```python
from build123d import *

# Parameters (mm, degrees)
EXTRUDE1_DEPTH                 = 2.515
M3X0_5_TAPPED_HOLE2_AT_2_COUNT = 2
M3X0_5_TAPPED_HOLE2_AT_2_PITCH = 37
M3X0_5_TAPPED_HOLE2_AT_3_COUNT = 2
M3X0_5_TAPPED_HOLE2_AT_3_PITCH = 74
M3X0_5_TAPPED_HOLE2_AT_4_COUNT = 2
M3X0_5_TAPPED_HOLE2_AT_4_PITCH = 111
M3X0_5_TAPPED_HOLE2_AT_5_COUNT = 2
M3X0_5_TAPPED_HOLE2_AT_5_PITCH = 148
CUT_EXTRUDE1_DEPTH             = 6.03
M3X0_5_TAPPED_HOLE1_D          = 3
M3X0_5_TAPPED_HOLE1_DEPTH      = 7.5
M3X0_5_TAPPED_HOLE1_TIP        = 0.901290929
F_2_5_2_5_DIAMETER_HOLE1_D     = 2.5
F_2_5_2_5_DIAMETER_HOLE1_DEPTH = 6
F_2_5_2_5_DIAMETER_HOLE1_TIP   = 0.751075774


with BuildPart() as part:
    # Sketch1 → Extrude1 (new body, symmetric)
    with BuildSketch(Plane.XY):
        with BuildLine():
            Line((29.232493618, 208), (4.5, 208))
            Line((4.5, 208), (4.5, 37.873672337))
            ThreePointArc((4.5, 37.873672337), (38.14007153, 0), (4.5, -37.873672337))
            Line((4.5, -37.873672337), (4.5, -208))
            Line((4.5, -208), (29.232493618, -208))
            Line((29.232493618, -208), (12, -85.384436669))
            Line((12, -85.384436669), (12, -60))
            ThreePointArc((12, -60), (14.850141486, -49.710084891), (22.588235294, -42.352941176))
            ThreePointArc((22.588235294, -42.352941176), (48, 0), (22.588235294, 42.352941176))
            ThreePointArc((22.588235294, 42.352941176), (14.850141486, 49.710084891), (12, 60))
            Line((12, 60), (12, 85.384436669))
            Line((12, 85.384436669), (29.232493618, 208))
        make_face()
    extrude(amount=EXTRUDE1_DEPTH, both=True)

    # Sketch32 → M3x0.5 Tapped Hole2 (revolve, cut)
    with BuildSketch(Plane(origin=(4.5, 198, 0), x_dir=(0, 0, 1), z_dir=(0, 1, 0))):
        Polygon((0, 0), (0, 8.401290929), (1.5, 7.5), (1.5, 0), align=None)
    m3x0_5_tapped_hole2 = revolve(axis=Axis((-1.85, 198, 0), (1, 0, 0)), mode=Mode.SUBTRACT)

    # M3x0.5 Tapped Hole2 at 2: M3x0.5 Tapped Hole2 ×2
    with Locations(*[(0, -i * M3X0_5_TAPPED_HOLE2_AT_2_PITCH, 0) for i in range(1, M3X0_5_TAPPED_HOLE2_AT_2_COUNT)]):
        add(m3x0_5_tapped_hole2, mode=Mode.SUBTRACT)

    # M3x0.5 Tapped Hole2 at 3: M3x0.5 Tapped Hole2 ×2
    with Locations(*[(0, -i * M3X0_5_TAPPED_HOLE2_AT_3_PITCH, 0) for i in range(1, M3X0_5_TAPPED_HOLE2_AT_3_COUNT)]):
        add(m3x0_5_tapped_hole2, mode=Mode.SUBTRACT)

    # M3x0.5 Tapped Hole2 at 4: M3x0.5 Tapped Hole2 ×2
    with Locations(*[(0, -i * M3X0_5_TAPPED_HOLE2_AT_4_PITCH, 0) for i in range(1, M3X0_5_TAPPED_HOLE2_AT_4_COUNT)]):
        add(m3x0_5_tapped_hole2, mode=Mode.SUBTRACT)

    # M3x0.5 Tapped Hole2 at 5: M3x0.5 Tapped Hole2 ×2
    with Locations(*[(0, -i * M3X0_5_TAPPED_HOLE2_AT_5_PITCH, 0) for i in range(1, M3X0_5_TAPPED_HOLE2_AT_5_COUNT)]):
        add(m3x0_5_tapped_hole2, mode=Mode.SUBTRACT)

    # Mirror2: M3x0.5 Tapped Hole2 across plane
    add(m3x0_5_tapped_hole2.mirror(Plane.ZX), mode=Mode.SUBTRACT)

    # Mirror2 copy 1 sketch → Mirror2 copy 1 (revolve, cut)
    with BuildSketch(Plane(origin=(4.5, -161, 0), x_dir=(0, 0, 1), z_dir=(0, -1, 0))):
        Polygon((0, 0), (0, -8.401290929), (1.5, -7.5), (1.5, 0), align=None)
    revolve(axis=Axis((-1.85, -161, 0), (-1, 0, 0)), mode=Mode.SUBTRACT)

    # Mirror2 copy 2 sketch → Mirror2 copy 2 (revolve, cut)
    with BuildSketch(Plane(origin=(4.5, -124, 0), x_dir=(0, 0, 1), z_dir=(0, -1, 0))):
        Polygon((0, 0), (0, -8.401290929), (1.5, -7.5), (1.5, 0), align=None)
    revolve(axis=Axis((-1.85, -124, 0), (-1, 0, 0)), mode=Mode.SUBTRACT)

    # Mirror2 copy 3 sketch → Mirror2 copy 3 (revolve, cut)
    with BuildSketch(Plane(origin=(4.5, -87, 0), x_dir=(0, 0, 1), z_dir=(0, -1, 0))):
        Polygon((0, 0), (0, -8.401290929), (1.5, -7.5), (1.5, 0), align=None)
    revolve(axis=Axis((-1.85, -87, 0), (-1, 0, 0)), mode=Mode.SUBTRACT)

    # Mirror2 copy 4 sketch → Mirror2 copy 4 (revolve, cut)
    with BuildSketch(Plane(origin=(4.5, -50, 0), x_dir=(0, 0, 1), z_dir=(0, -1, 0))):
        Polygon((0, 0), (0, -8.401290929), (1.5, -7.5), (1.5, 0), align=None)
    revolve(axis=Axis((-1.85, -50, 0), (-1, 0, 0)), mode=Mode.SUBTRACT)

    # Sketch36 → Cut-Extrude1 (cut, through all)
    with BuildSketch(Plane.XY.offset(2.515)):
        with BuildLine():
            Line((4.5, 193), (27.124381098, 193))
            Line((27.124381098, 193), (12, 85.384436669))
            Line((12, 85.384436669), (12, 60))
            ThreePointArc((12, 60), (14.850141486, 49.710084891), (22.588235294, 42.352941176))
            ThreePointArc((22.588235294, 42.352941176), (48, 0), (22.588235294, -42.352941176))
            ThreePointArc((22.588235294, -42.352941176), (14.850141486, -49.710084891), (12, -60))
            Line((12, -60), (12, -85.384436669))
            Line((12, -85.384436669), (29.232493618, -208))
            Line((29.232493618, -208), (4.5, -208))
            Line((4.5, -208), (4.5, -37.873672337))
            ThreePointArc((4.5, -37.873672337), (38.14007153, 0), (4.5, 37.873672337))
            Line((4.5, 37.873672337), (4.5, 193))
        make_face()
    extrude(amount=-CUT_EXTRUDE1_DEPTH, mode=Mode.SUBTRACT)

    # M3x0.5 Tapped Hole1
    with Locations(Plane(origin=(0, 208, 0), x_dir=(-1, 0, 0), z_dir=(0, 1, 0))):
        with Locations((-11, 0)):
            Hole(M3X0_5_TAPPED_HOLE1_D / 2, depth=M3X0_5_TAPPED_HOLE1_DEPTH)
            with Locations((0, 0, -(M3X0_5_TAPPED_HOLE1_DEPTH + M3X0_5_TAPPED_HOLE1_TIP / 2))):  # 118° drill point
                Cone(0, M3X0_5_TAPPED_HOLE1_D / 2, M3X0_5_TAPPED_HOLE1_TIP, mode=Mode.SUBTRACT)

    # 2.5 _2.5_ Diameter Hole1
    with Locations(Plane(origin=(0, 208, 0), x_dir=(-1, 0, 0), z_dir=(0, 1, 0))):
        with Locations((-22, 0)):
            Hole(F_2_5_2_5_DIAMETER_HOLE1_D / 2, depth=F_2_5_2_5_DIAMETER_HOLE1_DEPTH)
            with Locations((0, 0, -(F_2_5_2_5_DIAMETER_HOLE1_DEPTH + F_2_5_2_5_DIAMETER_HOLE1_TIP / 2))):  # 118° drill point
                Cone(0, F_2_5_2_5_DIAMETER_HOLE1_D / 2, F_2_5_2_5_DIAMETER_HOLE1_TIP, mode=Mode.SUBTRACT)


solid = part.part
```
Work out the finished part from the listing and answer in its coordinate system (mm). A direction names the side the tool comes from. Coordinates: 2 decimals unless noted, no trailing zeros. Order: outer loops, then holes, each group sorted by start corner. A loop starts at its lowest first (then second) coordinate and runs counter-clockwise, first axis right, second up. Notation, with made-up numbers: M 2.25,88.5 L 14.25,88.5 A17 cw 14.25,110.5 Z; hole C 18,-33.5 d5. An arc over 180 degrees is marked long. Use CSV: the item, a comma, the result in double quotes.
1) Section C-C on y = 205.75 is taken. Write down the section's boundary in (x, z) (3 decimals), plus the area to 3 significant figures.
Worked out:
outline,"M 4.5,-2.515 L 28.916,-2.515 L 28.916,2.515 L 4.5,2.515 Z; hole C 11,0 d3; hole C 22,0 d2.5"
area,"111 mm^2"
2) Determine the mould class of faces 1 (the face through (4.5, 201, 0)), 2 (the face through (12.745, 197.742, -0.034)), 3 (the face through (11.207, 199.755, -0.159)), 4 (the face through (28.164, 200.395, 0.035)) for opening direction Y: released by +Y, released by -Y, zero draft, split by the parting line, or undercut.
Worked out:
face 1,"zero draft"
face 2,"undercut"
face 3,"released by +Y"
face 4,"released by -Y"
3) Consider line 1 (Z direction, x = 22, y = 204.5) (3 decimals); line 2 (Z direction, x = 7, y = 198) (3 decimals); line 3 (X direction, y = 203, z = 0). Determine where each line is inside the solid, lowest interval first. Write a range as [from, to].
Worked out:
line 1,"z = [-2.515, -1.25], [1.25, 2.515]"
line 2,"z = [-2.515, -1.5], [1.5, 2.515]"
line 3,"x = [4.5, 9.5], [12.5, 20.75], [23.25, 28.53]"
4) Section A-A on x = 9 is taken. Write down the section's boundary in (y, z) (3 decimals).
Worked out:
outline,"M 193,-2.515 L 208,-2.515 L 208,2.515 L 193,2.515 Z; hole C 198,0 d3"
5) A flat-ended cylindrical pin translates along its axis: pin 1 Ø1.5 at (y, z) = (196, 1.5) entering from +X. Find the tip coordinate at first contact, or state that the pin passes through.
Worked out:
pin 1,"stops at x = 27.65"
6) Section B-B on y = 203.5 is taken. Write down the section's boundary in (x, z) (3 decimals).
Worked out:
outline,"M 4.5,-2.515 L 28.6,-2.515 L 28.6,2.515 L 4.5,2.515 Z; hole C 11,0 d3; hole C 22,0 d2.5"
7) For faces 5 (the face through (9.5, 204.2, 0.07)), 6 (the face through (17, 201, -2.515)), 7 (the face through (8.198, 196.513, -0.195)), determine the directions among +Z, -Z, +X, -X, +Y, -Y from which every point of the face is accessible in a straight line to the end or side of a thin tool.
Worked out:
face 5,"+Y"
face 6,"-Z, +X, -X, +Y, -Y"
face 7,"-X"
